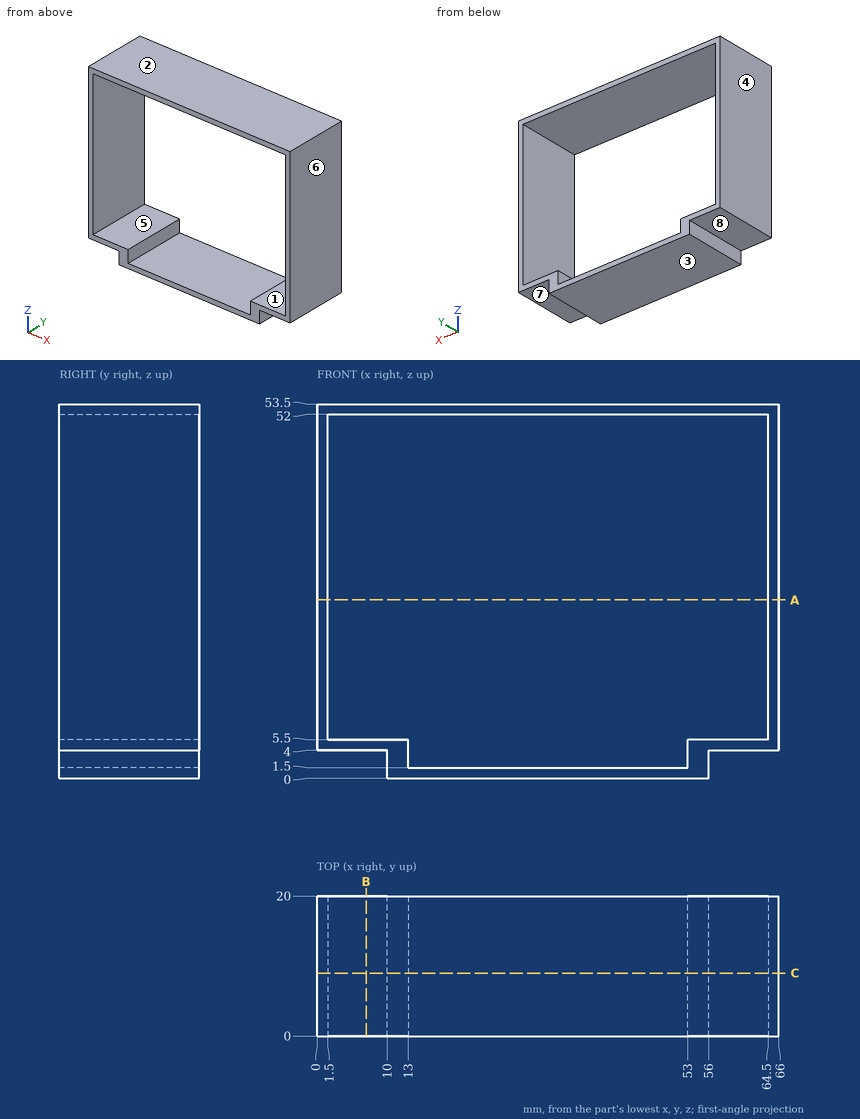
Can you work these out from the drawing? Everything is in mm from the part's minimum corner. A direction names the side the tool comes from. Give positions to 0.01 mm unless a question says otherwise; leave off trailing zeros. Loops run counter-clockwise (first coordinate to the right, second up) from the corner with the lowest first, then second, coordinate; pieces in that order, holes last. Notation, with made-up numbers: (54, 69.25) -> (112, 69.25) arc R19 ccw to (112, 92.25) -> close; hole circle Ø3 at (-20, -21.75). An arc over 180 degrees is marked (long way). Return JSON: item names as keys, results as strings.
Q1. I want a section at A-A, the plane z = 25.5. List the corners of the cut face in (x, y) for me.
Checks:
{"outline": "(0, 0) -> (1.5, 0) -> (1.5, 20) -> (0, 20) -> close; (64.5, 0) -> (66, 0) -> (66, 20) -> (64.5, 20) -> close"}
Q2. I want a section at C-C, the plane y = 9. List the corners of the cut face in (x, z) for me.
Checks:
{"outline": "(0, 4) -> (10, 4) -> (10, 0) -> (56, 0) -> (56, 4) -> (66, 4) -> (66, 53.5) -> (0, 53.5) -> close; hole (1.5, 5.5) -> (13, 5.5) -> (13, 1.5) -> (53, 1.5) -> (53, 5.5) -> (64.5, 5.5) -> (64.5, 52) -> (1.5, 52) -> close"}
Q3. For pin 1 Ø4.5 at (y, z) = (7, 1) entering from +X; pin 2 Ø5 at (x, y) = (3, 6) entering from -Z; pin 3 Ø3 at (y, z) = (6, 2) entering from -X, each with a flat end and sliding along its axis, tell me the tip position at first contact or that it passes through.
Checks:
{"pin 1": "stops at x = 56", "pin 2": "stops at z = 4", "pin 3": "stops at x = 10"}
Q4. On a 3-axis mill with a long thin cutter (end or side, diameter ignored), from which of +Z, -Z, +X, -X, +Y, -Y can I reach the whole of each face in a straight line? I mean the marked faces 5, 6, 7 and 8. Say none if no direction works.
Checks:
{"face 5": "+Y, -Y", "face 6": "+Z, -Z, +X, +Y, -Y", "face 7": "-Z, +X, +Y, -Y", "face 8": "-Z, -X, +Y, -Y"}
Q5. I need wall thicknesses on probe 1 along X at (y, z) = (17.25, 15.5); probe 2 along Z at (x, y) = (61, 14.75); probe 3 along Z at (x, y) = (22, 14). Which ranges of each line are inside material? Lowest first, please.
Checks:
{"probe 1": "x = 0 to 1.5, 64.5 to 66", "probe 2": "z = 4 to 5.5, 52 to 53.5", "probe 3": "z = 0 to 1.5, 52 to 53.5"}
Q6. I want a section at B-B, the plane x = 7. List the corners of the cut face in (y, z) for me.
Checks:
{"outline": "(0, 4) -> (20, 4) -> (20, 5.5) -> (0, 5.5) -> close; (0, 52) -> (20, 52) -> (20, 53.5) -> (0, 53.5) -> close"}
Q7. We'd pull the mould along Z, two halves only. Please class the marked faces 1, 2, 3 and 4: released by +Z, released by -Z, zero draft, split by the parting line, or undercut.
Checks:
{"face 1": "undercut", "face 2": "released by +Z", "face 3": "released by -Z", "face 4": "zero draft"}
